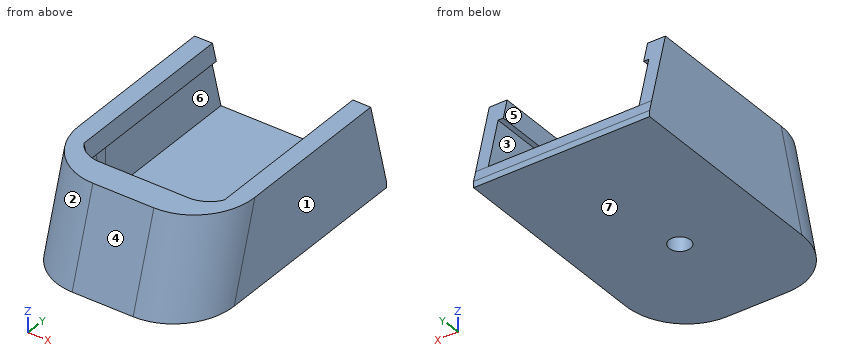
from build123d import *

# Parameters (mm, degrees)
F3_DEPTH    = 13
F4_DEPTH    = 12.2
F5_T1_DEPTH = 35.5
F6_DEPTH    = 15.3
F7_R        = 10
F8_DEPTH    = 28.5
F10_R       = 1.85
F11_DEPTH   = 5
F14_DEPTH   = 20


# Not quite as in the source:
# - a fillet or chamfer that OpenCascade refuses, or shapes differently, is made with other operations: its cross-section is extruded or revolved along the edge and cut away or added


with BuildPart() as f3:
    # F2 (on Right) → F3 (new body, symmetric)
    with BuildSketch(Plane.YZ):
        Polygon((-5.5, 3), (0, 3), (28, 3), (25.6314561435, 12.2), (-7.8685438565, 12.2), align=None)
    extrude(amount=F3_DEPTH, both=True)

    # F2 (on Right) → F4 (join, symmetric)
    with BuildSketch(Plane.YZ):
        Polygon((-8.7953653655, 15.8), (-7.8685438565, 12.2), (25.6314561435, 12.2), (24.7046346345, 15.8), align=None)
    extrude(amount=F4_DEPTH, both=True)

    # F5: fillet of radius 5.2 on 2 edges, made by hand

    # F5_s2 → F5_t1 (cut)
    with BuildSketch(Plane(origin=(0, -6.6759341801, 25.9309509046), x_dir=(1, 0, 0), z_dir=(0, 0.2493204059, -0.9684210526))):
        with BuildLine():
            ThreePointArc((7.8, 4.5783545716), (11.4769552622, 3.0553098338), (13, -0.6216454284))
            Line((13, -0.6216454284), (13, 4.5783545716))
            Line((13, 4.5783545716), (7.8, 4.5783545716))
        make_face()
        with BuildLine():
            ThreePointArc((-7.8, 4.5783545716), (-11.4769552622, 3.0553098338), (-13, -0.6216454284))
            Line((-13, -0.6216454284), (-13, 4.5783545716))
            Line((-13, 4.5783545716), (-7.8, 4.5783545716))
        make_face()
    extrude(amount=F5_T1_DEPTH, mode=Mode.SUBTRACT)


with BuildPart() as f6:
    # F1 (on Right) → F6 (new body, symmetric)
    with BuildSketch(Plane.YZ):
        Polygon((-18.7, 0), (0, 0), (0, 15.8), (-13.7, 15.8), align=None)
    extrude(amount=F6_DEPTH, both=True)

    # F7
    f7_edges = [f6.edges().sort_by_distance(p)[0] for p in [
        (15.3, -16.2, 7.9),
        (-15.3, -16.2, 7.9),
    ]]
    fillet(f7_edges, radius=F7_R)

    # F0 (on Front) → F8 (join)
    with BuildSketch(Plane.XZ):
        Polygon((-15.3, 0), (0, 0), (15.3, 0), (15.3, 15.8), (12.2, 15.8), (12.2, 12.2), (13.1, 12.2), (13.1, 3), (0, 3), (-13.1, 3), (-13.1, 12.2), (-12.2, 12.2), (-12.2, 15.8), (-15.3, 15.8), align=None)
    extrude(amount=-F8_DEPTH)

    # F9: cut F3
    add(f3.part, mode=Mode.SUBTRACT)


with BuildPart() as f11:
    # F10 (on Top) → F11 (new body)
    with BuildSketch(Plane.XY):
        Circle(F10_R)
    extrude(amount=F11_DEPTH)


with BuildPart() as f6_1:
    add(f6.part)

    # F12: cut F11
    add(f11.part, mode=Mode.SUBTRACT)

    # F13 (on Right) → F14 (cut, symmetric)
    with BuildSketch(Plane.YZ):
        Polygon((29.3071324871, 15.8), (24.7046346345, 15.8), (28, 3), (29.3071324871, -2.0772202713), align=None)
    extrude(amount=F14_DEPTH, both=True, mode=Mode.SUBTRACT)


solid = f6_1.part
Geometry: final body of the model. Coordinates: model frame, mm. Face numbers are marked on the shaded views. A direction names the side the tool comes from. Round coordinates to 2 decimals unless told otherwise and drop trailing zeros. Loops run counter-clockwise (first coordinate to the right, second up) from the corner with the lowest first, then second, coordinate; pieces in that order, holes last. Notation, with made-up numbers: (-16, 85.25) -> (-9, 85.25) arc R18 cw to (-9, 102.25) -> close; hole circle Ø10 at (32, -36). An arc over 180 degrees is marked (long way). One line per question, with ' | ' between items. Start each with the question number.
1. Section A-A on x = 0. Output: boundary loops of the cut face in (y, z).
2. Set-up query: the marked faces 5, 6 and 7. Return all of +Z, -Z, +X, -X, +Y, -Y with unobstructed straight access to the full face (end or side cutting, diameter ignored); none if empty.
3. Line query: line 1 along X through (y, z) = (0, 1.35); line 2 along X through (y, z) = (-1, 11); line 3 along Y through (x, z) = (0, 0.65). Output: solid intervals per line, ascending. Write a range as [from, to].
4. Section B-B on y = 18.5. Output: boundary loops of the cut face in (x, z).
5. Mould query, pull axis X, two halves, no side actions, for the marked faces 1, 2, 3 and 4. Classes: pulls with the +X half, pulls with the -X half, needs draft (parallel to the pull), parting line crosses it, or undercut.
6. Section C-C on x = 9. Output: boundary loops of the cut face in (y, z).
7. Contact query for flat-ended pins moving along their axis: pin 1 (1.5 mm diameter, centred on x = 2.5, z = 4, fed in from -Y); pin 2 (1 mm diameter, centred on x = 5.5, z = 9, fed in from -Y); pin 3 (5 mm diameter, centred on x = -1.5, z = 3.5, fed in from -Y); pin 4 (3 mm diameter, centred on x = 0, y = 0, fed in from +Z). Output: stop coordinate, or through.
Returned:
1) outline: (-18.7, 0) -> (-1.85, 0) -> (-1.85, 3) -> (-5.5, 3) -> (-8.8, 15.8) -> (-13.7, 15.8) -> close; (1.85, 0) -> (28.5, 0) -> (28.5, 1.06) -> (28, 3) -> (1.85, 3) -> close
2) face 5: +Z, +Y | face 6: +Y | face 7: -Z, +X, -X, +Y, -Y
3) line 1: x = [-15.3, -1.85], [1.85, 15.3] | line 2: x = [-15.3, -13], [13, 15.3] | line 3: y = [-18.49, -1.85], [1.85, 28.5]
4) outline: (-15.3, 0) -> (15.3, 0) -> (15.3, 15.8) -> (12.2, 15.8) -> (12.2, 12.2) -> (13.1, 12.2) -> (13.1, 3) -> (-13.1, 3) -> (-13.1, 12.2) -> (-12.2, 12.2) -> (-12.2, 15.8) -> (-15.3, 15.8) -> close
5) face 1: pulls with the +X half | face 2: pulls with the -X half | face 3: undercut | face 4: needs draft
6) outline: (-17.96, 0) -> (28.5, 0) -> (28.5, 1.06) -> (28, 3) -> (-5.36, 3) -> (-8.65, 15.8) -> (-12.96, 15.8) -> close
7) pin 1: stops at y = -17.67 | pin 2: stops at y = -16.01 | pin 3: stops at y = -18.38 | pin 4: passes through
